```python
from build123d import *

# Parameters (mm, degrees)
SKETCH1_R           = 1.73
BOSS_EXTRUDE1_DEPTH = 2


with BuildPart() as part:
    # Sketch1 → Boss-Extrude1 (new body, symmetric)
    with BuildSketch(Plane.XY):
        with BuildLine():
            Line((-17.141234423, -7.500996555), (-3.621301313, -9.563286323))
            Line((-3.621301313, -9.563286323), (-5.418135156, -8.404987295))
            ThreePointArc((-5.418135156, -8.404987295), (-9.351968753, 3.541282315), (1.507927798, 9.885653937))
            Line((1.507927798, 9.885653937), (-14.125378827, 12.270311319))
            ThreePointArc((-14.125378827, 12.270311319), (-25.518960562, 3.89258518), (-17.141234423, -7.500996555))
        make_face()
        with Locations((-15.633306625, 2.384657382)):
            Circle(SKETCH1_R, mode=Mode.SUBTRACT)
        with BuildLine():
            Line((-3.621301313, -9.563286323), (-1.507927798, -9.885653937))
            ThreePointArc((-1.507927798, -9.885653937), (9.351968753, -3.541282315), (5.418135156, 8.404987295))
            ThreePointArc((5.418135156, 8.404987295), (3.541282315, 9.351968753), (1.507927798, 9.885653937))
            ThreePointArc((1.507927798, 9.885653937), (-9.351968753, 3.541282315), (-5.418135156, -8.404987295))
            Line((-5.418135156, -8.404987295), (-3.621301313, -9.563286323))
        make_face()
        Circle(SKETCH1_R, mode=Mode.SUBTRACT)
        with BuildLine():
            ThreePointArc((5.418135156, 8.404987295), (9.351968753, -3.541282315), (-1.507927798, -9.885653937))
            Line((-1.507927798, -9.885653937), (-3.621301313, -9.563286323))
            Line((-3.621301313, -9.563286323), (49.686174905, -43.927063542))
            ThreePointArc((49.686174905, -43.927063542), (63.509297356, -40.940211402), (60.522445216, -27.117088952))
            Line((60.522445216, -27.117088952), (5.418135156, 8.404987295))
        make_face()
    extrude(amount=BOSS_EXTRUDE1_DEPTH, both=True)


solid = part.part
```
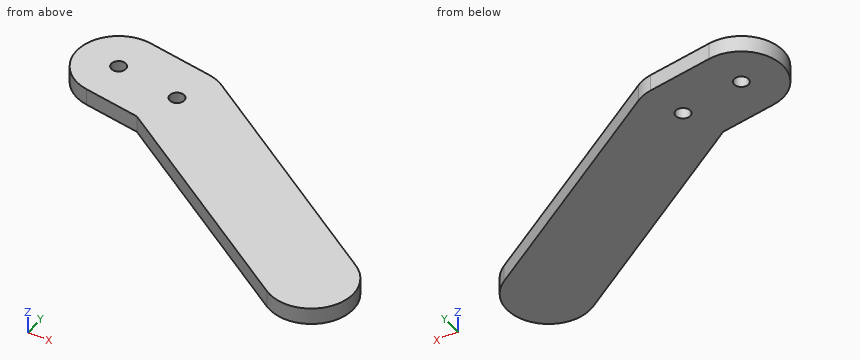
The listing builds one solid part. Answer for the finished solid, in the listing's coordinates (mm). Coordinates: 2 decimals unless noted, no trailing zeros. Write each loop counter-clockwise with the first axis right and the second up, starting at its lowest first coordinate (ties: lowest second). Pieces come first, ordered by that corner, then holes.
Q1. Section A-A, the plane z = -0.4 is taken. Write down the section's boundary in (x, y), then the cut area to 3 significant figures.
Returned:
outline: (-17.14, -7.5) - (-3.62, -9.56) - (49.69, -43.93) arc R10 ccw to (60.52, -27.12) - (5.42, 8.4) arc R10 ccw to (1.51, 9.89) - (-14.13, 12.27) arc R10 ccw to start; hole circle Ø3.46 at (-15.63, 2.38); hole circle Ø3.46 at (0, 0)
area: 1,920 mm2
Q2. Given P1, Ø2, axis at y = -2.5, z = 1.5, coming from the +X side; P2, Ø2, axis at x = 38, z = -1, coming from the +Y side; P3, Ø1, axis at y = -15.5, z = -0.5, coming from the -X side, each flat-ended and moving along its own axis, determine where each tip first touches the part or whether it passes through.
Returned:
P1: stops at x = 23.89
P2: stops at y = -11.95
P3: stops at x = 4.81
Q3. Section B-B, the plane x = 0 is taken. Write down the section's boundary in (y, z), then the cut area to 3 significant figures.
Returned:
outline: (-11.9, -2) - (-1.73, -2) - (-1.73, 2) - (-11.9, 2) - close; (1.73, -2) - (10.12, -2) - (10.12, 2) - (1.73, 2) - close
area: 74.2 mm2
Q4. Find the intervals of material crossed by line 1 along X through (y, z) = (-1, 1.3); line 2 along X through (y, z) = (-28.5, 0.7); line 3 along Y through (x, z) = (50.5, -1.6), in increasing order.
Returned:
line 1: x = -25.04 to -1.41, 1.41 to 20.01
line 2: x = 25.75 to 62.22
line 3: y = -44.4 to -20.66
Q5. Section C-C, the plane y = -18.5 is taken. Write down the section's boundary in (x, z), then the cut area to 3 significant figures.
Returned:
outline: (10.24, -2) - (47.16, -2) - (47.16, 2) - (10.24, 2) - close
area: 148 mm2
Q6. Section D-D, the plane x = 39.5 is taken. Write down the section's boundary in (y, z).
Returned:
outline: (-37.36, -2) - (-13.57, -2) - (-13.57, 2) - (-37.36, 2) - close
